Source: three-view drawing plus pictorial views. Frame: mm from the lowest corner of the part. A direction names the side the tool comes from. Give positions to 0.01 mm unless a question says otherwise; leave off trailing zeros. Write each loop counter-clockwise with the first axis right and the second up, starting at its lowest first coordinate (ties: lowest second). Pieces come first, ordered by that corner, then holes.
Q1. Cut plane B-B on y = 37.5. Return the cut outline in (x, z).
Q2. Cut plane C-C on z = 36.5. Return the cut outline in (x, y), plus the area to 3 significant figures.
Q3. Cut plane A-A on x = 5.5. Return the cut outline in (y, z), plus the area to 3 significant figures.
Q4. Line query: L1, parallel to X at y = 17, z = 5.5; L2, parallel to X at y = 23, z = 5; L3, parallel to Z at x = 37.5, y = 6. Output: solid intervals per line, ascending.
Q5. Pin query (flat end, axial travel): pin 1 (8 mm diameter, centred on x = 33.5, z = 12.5, fed in from +Y); pin 2 (12.5 mm diameter, centred on x = 14.5, z = 29.5, fed in from +Y). Return the tip coordinate at first contact, or that it passes through.
Q6. Cut plane D-D on x = 21. Return the cut outline in (y, z), plus the area to 3 significant figures.
Q7. Reachability of the marked faces 1 and 2 from +Z, -Z, +X, -X, +Y, -Y: full face, straight path, thin tool, end or side. Return the list, or none.
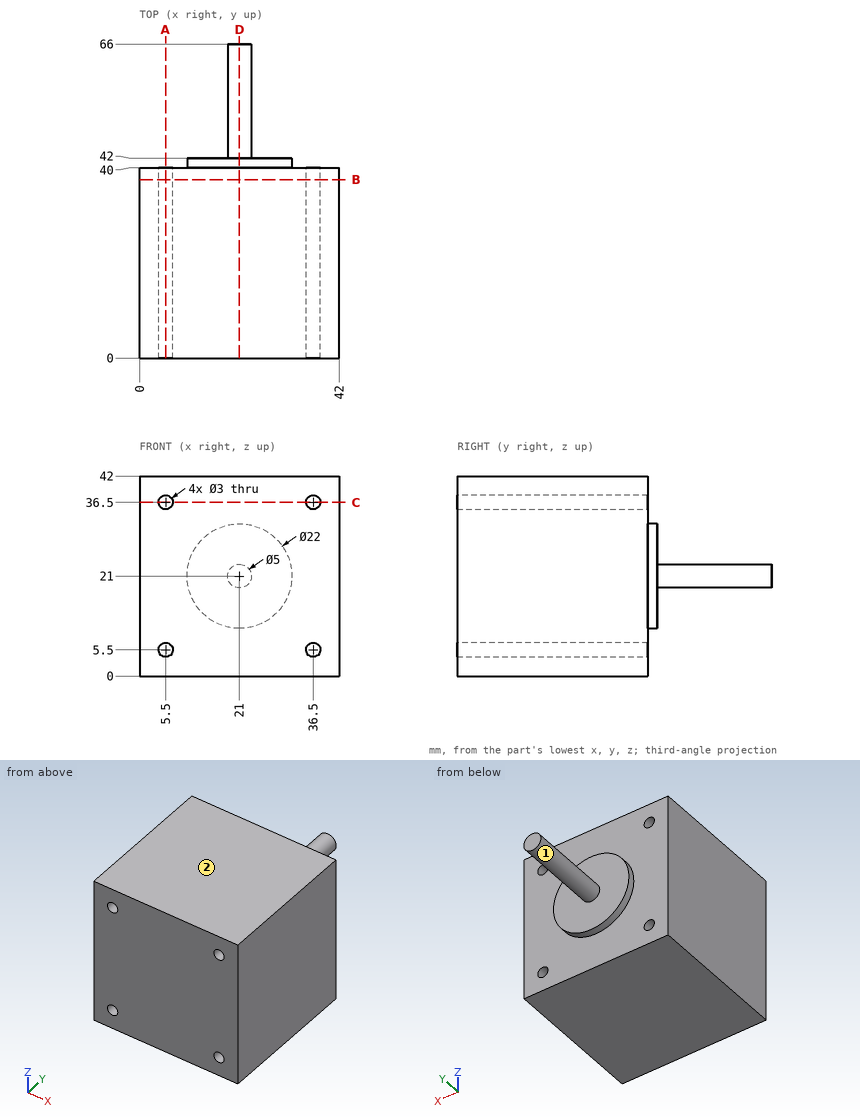
Data:
1. outline: (0, 0) - (42, 0) - (42, 42) - (0, 42) - close; hole circle Ø3 at (5.5, 5.5); hole circle Ø3 at (5.5, 36.5); hole circle Ø3 at (36.5, 5.5); hole circle Ø3 at (36.5, 36.5)
2. outline: (0, 0) - (4, 0) - (4, 40) - (0, 40) - close; (7, 0) - (35, 0) - (35, 40) - (7, 40) - close; (38, 0) - (42, 0) - (42, 40) - (38, 40) - close
2. area: 1,440 mm2
3. outline: (0, 0) - (40, 0) - (40, 4) - (0, 4) - close; (0, 7) - (40, 7) - (40, 35) - (0, 35) - close; (0, 38) - (40, 38) - (40, 42) - (0, 42) - close
3. area: 1,440 mm2
4. L1: x = 0 to 4, 7 to 35, 38 to 42
4. L2: x = 0 to 4.09, 6.91 to 35.09, 37.91 to 42
4. L3: z = 0 to 4.38, 6.62 to 35.38, 37.62 to 42
5. pin 1: stops at y = 40
5. pin 2: stops at y = 42
6. outline: (0, 0) - (40, 0) - (40, 10) - (42, 10) - (42, 18.5) - (66, 18.5) - (66, 23.5) - (42, 23.5) - (42, 32) - (40, 32) - (40, 42) - (0, 42) - close
6. area: 1,840 mm2
7. face 1: +Y
7. face 2: +Z, +X, -X, +Y, -Y
